The drawing under review shows one solid part. Ordinate dimensions are in mm from its lowest x, y, z. A direction names the side the tool comes from. Give positions to 0.01 mm unless a question says otherwise; leave off trailing zeros. Order: outer loops, then holes, each group sorted by start corner. A loop starts at its lowest first (then second) coordinate and runs counter-clockwise, first axis right, second up. Notation, with made-up numbers: (-12.75, -10) - (8.25, -10) arc R21 ccw to (8.25, 27) - close; hole circle Ø11 at (60, 82). An arc over 180 degrees is marked (long way). Answer as a JSON object with one key per item and string values. Group by question number.
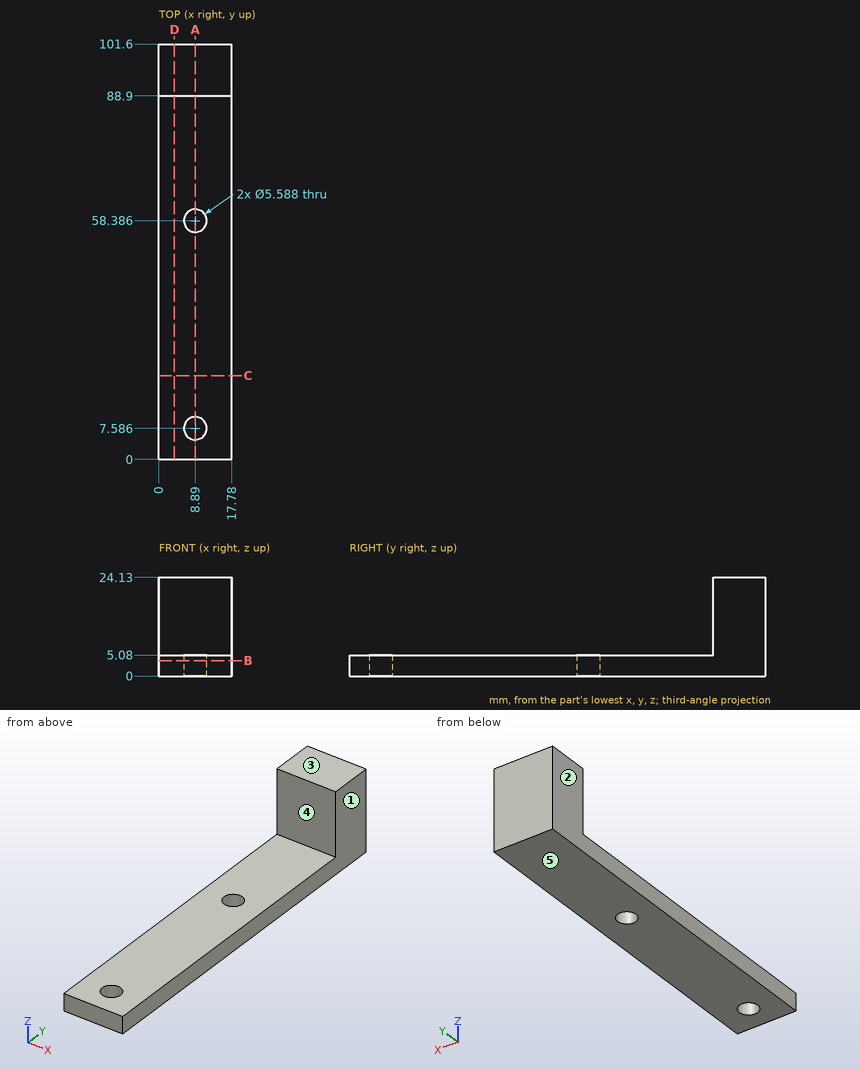
1) Consider section C-C (y = 20.5). Give the boundary of the cut face in (x, z).
2) For pin 1 (9 mm diameter, centred on x = 6.5, y = 53.5, fed in from +Z); pin 2 (8 mm diameter, centred on x = 14.5, z = 18, fed in from -Y); pin 3 (3.5 mm diameter, centred on x = 8.89, y = 7.59, fed in from +Z), all flat-tipped, find the tip position at first contact; note any pin that passes through.
3) Consider section D-D (x = 3.75). Give the boundary of the cut face in (y, z), plus the area to 3 significant figures.
4) Mouldability with a two-part tool opening along X and no side actions: class the marked faces 1, 2 and 3 as released by +X, released by -X, zero draft, split by the parting line, or undercut.
5) Consider section B-B (z = 3.75). Give the boundary of the cut face in (x, y).
6) Consider section A-A (x = 8.89). Give the boundary of the cut face in (y, z), plus the area to 3 significant figures.
7) For the marked faces 4 and 5, list the 3-axis set-ups (+Z, -Z, +X, -X, +Y, -Y) from which the entire face can be reached by the end or side of a thin tool; tool diameter is ignored.
8) For line 1 (Y direction, x = 8.89, z = 1.95); line 2 (Z direction, x = 8.5, y = 68); line 3 (Y direction, x = 6.5, z = 4) (1 decimal), list the stretches that pass through material, from the lowest coordinate up.
Result set:
{
 "1": {"outline": "(0, 0) - (17.78, 0) - (17.78, 5.08) - (0, 5.08) - close"},
 "2": {"pin 1": "stops at z = 5.08", "pin 2": "stops at y = 88.9", "pin 3": "passes through"},
 "3": {"outline": "(0, 0) - (101.6, 0) - (101.6, 24.13) - (88.9, 24.13) - (88.9, 5.08) - (0, 5.08) - close", "area": "758 mm2"},
 "4": {"face 1": "released by +X", "face 2": "released by -X", "face 3": "zero draft"},
 "5": {"outline": "(0, 0) - (17.78, 0) - (17.78, 101.6) - (0, 101.6) - close; hole circle Ø5.59 at (8.89, 7.59); hole circle Ø5.59 at (8.89, 58.39)"},
 "6": {"outline": "(0, 0) - (4.79, 0) - (4.79, 5.08) - (0, 5.08) - close; (10.38, 0) - (55.59, 0) - (55.59, 5.08) - (10.38, 5.08) - close; (61.18, 0) - (101.6, 0) - (101.6, 24.13) - (88.9, 24.13) - (88.9, 5.08) - (61.18, 5.08) - close", "area": "701 mm2"},
 "7": {"face 4": "+Z, +X, -X, -Y", "face 5": "-Z, +X, -X, +Y, -Y"},
 "8": {"line 1": "y = 0 to 4.79, 10.38 to 55.59, 61.18 to 101.6", "line 2": "z = 0 to 5.08", "line 3": "y = 0 to 6.1, 9 to 56.9, 59.8 to 101.6"}
}
